Work out the finished part from the listing and answer in its coordinate system (mm). A direction names the side the tool comes from. Coordinates: 2 decimals unless noted, no trailing zeros. Write each loop counter-clockwise with the first axis right and the second up, starting at its lowest first coordinate (ties: lowest second). Pieces come first, ordered by that corner, then holes. Notation, with made-up numbers: (-37.75, -26.75) - (21.25, -26.75) arc R22 cw to (21.25, 5.25) - close; hole circle Ø3 at (-29.75, 19). An arc over 180 degrees is marked (long way). One line per item, written item: value.
```python
from build123d import *

# Parameters (mm, degrees)
F0_W          = 10
F0_H          = 10
F0_R          = 3.25
F1_DEPTH      = 10
F0_H_2        = 5
F2_DEPTH      = 10
F3_R          = 4.25
F3_R_2        = 3.25
F4_DEPTH      = 10
F5_R          = 1.5
F6_DEPTH      = 5.001
F6_DEPTH_BACK = 5.001
F7_R          = 2.5
F8_DEPTH      = 10


with BuildPart() as f1:
    # F0 (on Front) → F1 (new body)
    with BuildSketch(Plane.XZ):
        Rectangle(F0_W, F0_H)
        Circle(F0_R, mode=Mode.SUBTRACT)
    extrude(amount=-F1_DEPTH)

    # F0 (on Front) → F2 (join)
    with BuildSketch(Plane.XZ):
        with Locations((0, 7.5)):
            Rectangle(F0_W, F0_H_2)
        Rectangle(F0_W, F0_H)
        Circle(F0_R, mode=Mode.SUBTRACT)
    extrude(amount=F2_DEPTH)

    # F3 (on face) → F4 (cut)
    with BuildSketch(Plane(origin=(0, 10, 0), x_dir=(-1, 0, 0), z_dir=(0, 1, 0))):
        Circle(F3_R)
        Circle(F3_R_2, mode=Mode.SUBTRACT)
        Circle(F3_R_2)
    extrude(amount=-F4_DEPTH, mode=Mode.SUBTRACT)

    # F5 (on Right) → F6 (cut, two sides)
    with BuildSketch(Plane.YZ) as f6_sk:
        with Locations((-3.5, 4.5)):
            Circle(F5_R)
    extrude(amount=-F6_DEPTH, mode=Mode.SUBTRACT)
    extrude(f6_sk.sketch, amount=F6_DEPTH_BACK, mode=Mode.SUBTRACT)

    # F7 (on face) → F8 (cut)
    with BuildSketch(Plane.XY.offset(10)):
        with Locations((0, -3.5)):
            Circle(F7_R)
    extrude(amount=-F8_DEPTH, mode=Mode.SUBTRACT)


solid = f1.part
```
Item 1: Section B-B, the plane z = 0 is taken. Determine the outline of the cut face in (x, y), then the cut area to 3 significant figures.
Evaluation:
outline: (-5, -10) - (-3.25, -10) - (-3.25, 0) - (-4.25, 0) - (-4.25, 10) - (-5, 10) - close; (3.25, -10) - (5, -10) - (5, 10) - (4.25, 10) - (4.25, 0) - (3.25, 0) - close
area: 50.0 mm2
Item 2: Section D-D, the plane x = 4 is taken. Determine the outline of the cut face in (y, z).
Evaluation:
outline: (-10, -5) - (10, -5) - (10, -1.44) - (0, -1.44) - (0, 1.44) - (10, 1.44) - (10, 5) - (0, 5) - (0, 10) - (-10, 10) - close; hole circle Ø3 at (-3.5, 4.5)
Item 3: Determine the mould class of faces 1 (the face through (0, -10, 4)), 2 (the face through (-1, -6, 10)), 3 (the face through (-0.705, -4.93, -3.173)) for opening direction Z: +Z half, -Z half, draft (parallel to the pull), parting line (faces both ways), or undercut.
Evaluation:
face 1: draft
face 2: +Z half
face 3: undercut
Item 4: Section A-A, the plane x = 0 is taken. Determine the outline of the cut face in (y, z).
Evaluation:
outline: (-10, -5) - (10, -5) - (10, -4.25) - (0, -4.25) - (0, -3.25) - (-10, -3.25) - close; (-10, 3.25) - (-6, 3.25) - (-6, 10) - (-10, 10) - close; (-1, 3.25) - (0, 3.25) - (0, 4.25) - (10, 4.25) - (10, 5) - (0, 5) - (0, 10) - (-1, 10) - close
Item 5: Section C-C, the plane y = -3.5 is taken. Determine the outline of the cut face in (x, z), then the cut area to 3 significant figures.
Evaluation:
outline: (-5, -5) - (5, -5) - (5, 3) - (2.5, 3) - (2.5, 2.08) arc R3.25 cw (long way) to (-2.5, 2.08) - (-2.5, 3) - (-5, 3) - close; (-5, 6) - (-2.5, 6) - (-2.5, 10) - (-5, 10) - close; (2.5, 6) - (5, 6) - (5, 10) - (2.5, 10) - close
area: 66.3 mm2
Item 6: Consider probe 1 along Z at (x, y) = (-3.5, -3.5); probe 2 along Z at (x, y) = (0, 2.5); probe 3 along X at (y, z) = (-3.5, 9.75). Determine where each line is inside the solid, lowest interval first.
Evaluation:
probe 1: z = -5 to 3, 6 to 10
probe 2: z = -5 to -4.25, 4.25 to 5
probe 3: x = -5 to -2.5, 2.5 to 5
Item 7: Which of the six approach directions +Z, -Z, +X, -X, +Y, -Y give full straight-line access (tool end or side, diameter ignored) to faces 4 (the face through (0, 0, -5)), 5 (the face through (0, 5, 5)), 6 (the face through (-2.285, 5.07, 3.584)), 7 (the face through (-2.5, -3.4, 7))?
Evaluation:
face 4: -Z, +X, -X, +Y, -Y
face 5: +Z, +X, -X, +Y
face 6: +Y
face 7: +Z
Item 8: Given pin 1 (5 mm diameter, centred on x = 0, z = 0, fed in from -Y); pin 2 (4 mm diameter, centred on x = 0.5, z = -1.5, fed in from +Y); pin 3 (1.5 mm diameter, centred on x = 1, y = 5.5, fed in from +Z), each flat-ended and moving along its own axis, determine where each tip first touches the part or whether it passes through.
Evaluation:
pin 1: passes through
pin 2: stops at y = 0
pin 3: stops at z = 5
